The listing builds one solid part. Answer for the finished solid, in the listing's coordinates (mm). A direction names the side the tool comes from. Round coordinates to 2 decimals unless told otherwise and drop trailing zeros. Order: outer loops, then holes, each group sorted by start corner. A loop starts at its lowest first (then second) coordinate and runs counter-clockwise, first axis right, second up. Notation, with made-up numbers: M 53.25,-19 L 93.25,-19 A27 cw 93.25,4 Z; hole C 87,80 d7. An arc over 180 degrees is marked long. Write item = value, one per line. Start each with the question number.
(1) A cutting plane is placed at C-C, the plane x = 15. Determine the outline of the cut face in (y, z), and give its area (3 significant figures).
(2) A cutting plane is placed at A-A, the plane y = 15. Determine the outline of the cut face in (x, z), and give its area (3 significant figures).
(3) A cutting plane is placed at B-B, the plane z = 10. Determine the outline of the cut face in (x, y).
(4) Straight lines are drawn through the part: probe 1 along Y at (x, z) = (15, 9.5); probe 2 along Y at (x, z) = (-21.5, 9.5); probe 3 along Y at (x, z) = (-9, 4.5). For each, find the intervals that lie inside material, in ascending order. Write a range as from..to.
(5) For a pull along X with two mould halves and no side action, classify faces 1 (the face through (-9, -11, 6)), 2 (the face through (30, 0, 12)), 3 (the face through (0, -22, 5)) as released by +X, released by -X, zero draft, split by the parting line, or undercut.
(6) Which of the six approach directions +Z, -Z, +X, -X, +Y, -Y give full straight-line access (tool end or side, diameter ignored) to faces 4 (the face through (-9, 17, 6)), 5 (the face through (0, -25, 15)), 6 (the face through (0, -19, 3))?
(7) A cutting plane is placed at D-D, the plane x = -3.5. Determine the outline of the cut face in (y, z), and give its area (3 significant figures).
(8) Each of these flat-tipped pins is pushed along its axis until it touches: pin 1 (3.5 mm diameter, centred on x = 15, y = 15, fed in from -Z); pin 2 (5.5 mm diameter, centred on x = 6.5, z = 2, fed in from -Y); pin 3 (8.5 mm diameter, centred on x = -6.5, y = 0.5, fed in from -Z); pin 4 (1.8 mm diameter, centred on x = 2.5, y = -23, fed in from -Z). Where does it stop, or does it pass through?
from build123d import *

# Parameters (mm, degrees)
F0_W     = 60
F0_H     = 50
F0_R     = 2.75
F1_DEPTH = 25
F2_W     = 60
F2_H     = 5
F3_DEPTH = 6
F4_R     = 5
F5_W     = 27
F5_H     = 28
F6_DEPTH = 17
F7_R     = 5


with BuildPart() as f1:
    # F0 (on Top) → F1 (new body)
    with BuildSketch(Plane.XY):
        Rectangle(F0_W, F0_H)
        with Locations((15, -15)):
            Circle(F0_R, mode=Mode.SUBTRACT)
        with Locations((15, 15)):
            Circle(F0_R, mode=Mode.SUBTRACT)
    extrude(amount=F1_DEPTH)

    # F2 (on face) → F3 (cut)
    with BuildSketch(Plane.XZ.offset(25)):
        with Locations((0, 2.5)):
            Rectangle(F2_W, F2_H)
    extrude(amount=-F3_DEPTH, mode=Mode.SUBTRACT)

    # F4
    f4_edges = [f1.edges().sort_by_distance(p)[0] for p in [
        (30, -25, 15),
        (-30, -25, 15),
        (-30, 25, 12.5),
        (30, 25, 12.5),
    ]]
    fillet(f4_edges, radius=F4_R)

    # F5 (on face) → F6 (cut)
    with BuildSketch(Plane(origin=(0, 0, 0), x_dir=(1, 0, 0), z_dir=(0, 0, -1))):
        with Locations((-8.5, -3)):
            Rectangle(F5_W, F5_H)
    extrude(amount=-F6_DEPTH, mode=Mode.SUBTRACT)

    # F7
    f7_edges = [f1.edges().sort_by_distance(p)[0] for p in [
        (-8.5, -11, 17),
        (5, 3, 17),
        (-8.5, 17, 17),
        (-22, 3, 17),
    ]]
    fillet(f7_edges, radius=F7_R)


solid = f1.part
Reported:
q1.outline = M -25,5 L -19,5 L -19,0 L -17.75,0 L -17.75,25 L -25,25 Z; M -12.25,0 L 12.25,0 L 12.25,25 L -12.25,25 Z; M 17.75,0 L 25,0 L 25,25 L 17.75,25 Z
q1.area = 945 mm²
q2.outline = M -30,0 L -22,0 L -22,12 A5 cw -20,16 L 3,16 A5 cw 5,12 L 5,0 L 12.25,0 L 12.25,25 L -30,25 Z; M 17.75,0 L 30,0 L 30,25 L 17.75,25 Z
q2.area = 935 mm²
q3.outline = M -30,-20 A5 ccw -25,-25 L 25,-25 A5 ccw 30,-20 L 30,20 A5 ccw 25,25 L -25,25 A5 ccw -30,20 Z; hole M -22,-11 L 5,-11 L 5,17 L -22,17 Z; hole C 15,-15 d5.5; hole C 15,15 d5.5
q4.probe_1 = -25..-17.75, -12.25..12.25, 17.75..25
q4.probe_2 = -25..-11, 17..25
q4.probe_3 = -19..-11, 17..25
q5.face_1 = undercut
q5.face_2 = released by +X
q5.face_3 = zero draft
q6.face_4 = -Z
q6.face_5 = +Z, -Z, +X, -X, -Y
q6.face_6 = -Z, +X, -X, -Y
q7.outline = M -25,5 L -19,5 L -19,0 L -11,0 L -11,12 A5 cw -6,17 L 12,17 A5 cw 17,12 L 17,0 L 25,0 L 25,25 L -25,25 Z
q7.area = 755 mm²
q8.pin_1 = through
q8.pin_2 = -19
q8.pin_3 = 17
q8.pin_4 = 5
